Geometry check sheet. Reference: drawing and pictorial views, mm from the part's lowest x, y, z. A direction names the side the tool comes from. Round coordinates to 2 decimals unless told otherwise and drop trailing zeros. Loops run counter-clockwise (first coordinate to the right, second up) from the corner with the lowest first, then second, coordinate; pieces in that order, holes last. Notation, with made-up numbers: (76, 53) - (127, 53) arc R7 ccw to (127, 60) - close; hole circle Ø2 at (2.25, 29.5). An arc over 180 degrees is marked (long way). Put each result on its own line as item: value. Start each with the question number.
Item 1: Tool access check on the marked faces 1, 2, 3 and 4. Record the directions out of +Z, -Z, +X, -X, +Y, -Y that give a thin tool (end or side, any length) a straight path to the whole face; none if there is none.
Item 2: Section check D-D, the plane x = 50.5. Record the cut outline in (y, z), and give its area (3 significant figures).
Item 3: Gauge pin test, flat ends, axial feed: pin 1 Ø8 at (y, z) = (69, 21) entering from +X; pin 2 Ø5 at (y, z) = (70.5, 36.5) entering from -X; pin 3 Ø1 at (x, y) = (17, 64) entering from -Z; pin 4 Ø11 at (x, y) = (7, 70) entering from +Z. Record the tip position at first contact, or that the pin passes through.
Item 4: Section check B-B, the plane z = 17. Record the cut outline in (x, y), and give its area (3 significant figures).
Item 5: Material ranges on line 1 along Y through (x, z) = (75.5, 41); line 2 along Z through (x, y) = (61, 87); line 3 along Y through (x, z) = (52, 24), recorded low to high.
Item 6: Section check A-A, the plane x = 83.5. Record the cut outline in (y, z), and give its area (3 significant figures).
Item 7: Draft check along Y on the marked faces 5, 6, 7 and 8. Enter one of: pulls with the +Y half, pulls with the -Y half, needs draft (parallel to the pull), parting line crosses it, or undercut.
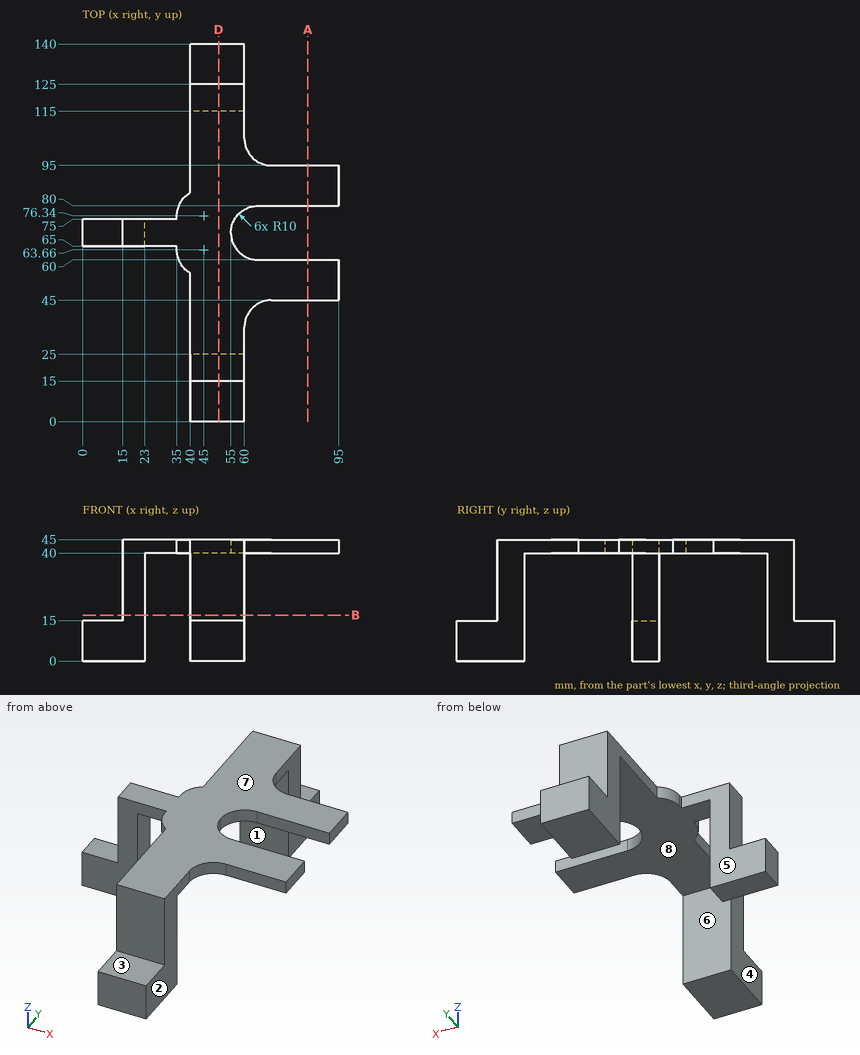
Check result:
1. face 1: -Z, +X, -X
1. face 2: +Z, -Z, +X, -Y
1. face 3: +Z, +X, -X, -Y
1. face 4: +Z, -Z, -X, -Y
2. outline: (0, 0) - (25, 0) - (25, 40) - (115, 40) - (115, 0) - (140, 0) - (140, 15) - (125, 15) - (125, 45) - (15, 45) - (15, 15) - (0, 15) - close
2. area: 1,800 mm²
3. pin 1: x = 23
3. pin 2: x = 15
3. pin 3: through
3. pin 4: z = 15
4. outline: (15, 65) - (23, 65) - (23, 75) - (15, 75) - close; (40, 15) - (60, 15) - (60, 25) - (40, 25) - close; (40, 115) - (60, 115) - (60, 125) - (40, 125) - close
4. area: 480 mm²
5. line 1: 45 to 60, 80 to 95
5. line 2: 40 to 45
5. line 3: 15 to 25, 115 to 125
6. outline: (45, 40) - (60, 40) - (60, 45) - (45, 45) - close; (80, 40) - (95, 40) - (95, 45) - (80, 45) - close
6. area: 150 mm²
7. face 5: pulls with the +Y half
7. face 6: undercut
7. face 7: needs draft
7. face 8: undercut
